Design review of the part built by this model. Coordinates are the model's own, in mm. Coordinates: 2 decimals unless noted, no trailing zeros. Loops run counter-clockwise (first coordinate to the right, second up) from the corner with the lowest first, then second, coordinate; pieces in that order, holes last. Notation, with made-up numbers: M 67.25,-5 L 108.25,-5 A20 ccw 108.25,27 Z; hole C 55.25,20.5 d2. An arc over 180 degrees is marked long. Answer as a JSON object with one key per item and string values. Group by question number.
1. Insertion check: pin 1 (4 mm diameter, centred on x = 64, z = 8.5, fed in from -Y); pin 2 (3.5 mm diameter, centred on y = -17, z = 7.5, fed in from -X) (3 decimals); pin 3 (0.5 mm diameter, centred on x = -104.5, y = -19, fed in from -Z). Each pin has a flat end and moves straight along its axis. Give the tip position at first contact, or say it passes through.
2. To check wall thickness, follow probe 1 along X at (y, z) = (-35, 7) (3 decimals); probe 2 along X at (y, z) = (-9.5, 2) (3 decimals); probe 3 along Y at (x, z) = (-87.5, 7) (1 decimal). State the ranges of each line that lie inside material, in increasing order.
3. Consider section A-A (z = 3.75). State the section outline as (x, y) points (3 decimals), then the cut area to 3 significant figures.
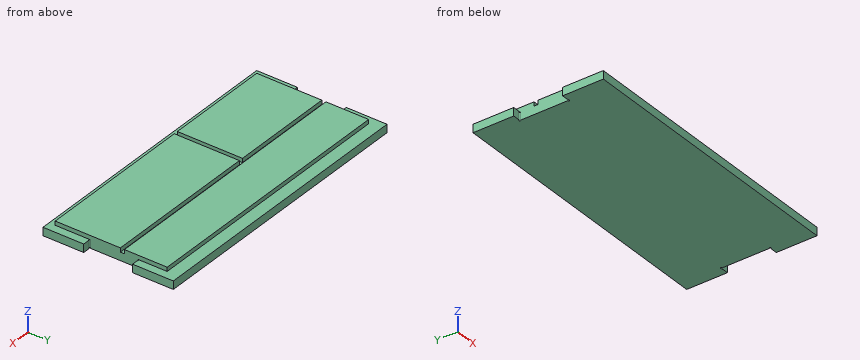
from build123d import *

# Parameters (mm, degrees)
F0_W     = 222.25
F0_H     = 101.6
F1_DEPTH = 9.525
F2_W     = 6.35
F2_H     = 38.1
F3_DEPTH = 9.526
F5_DEPTH = 3.175
F6_W     = 3.175
F6_H     = 50.8
F7_DEPTH = 3.175
F9_DEPTH = 6.35


with BuildPart() as f1:
    # F0 (on Top) → F1 (new body)
    with BuildSketch(Plane.XY):
        Rectangle(F0_W, F0_H)
    extrude(amount=F1_DEPTH)

    # F2 (on face) → F3 (cut, through all)
    with BuildSketch(Plane.XY.offset(9.525)):
        with Locations((-107.95, 0)):
            Rectangle(F2_W, F2_H)
        with Locations((107.95, 0)):
            Rectangle(F2_W, F2_H)
    extrude(amount=-F3_DEPTH, mode=Mode.SUBTRACT)

    # F4 (on face) → F5 (cut)
    with BuildSketch(Plane.XY.offset(9.525)):
        Polygon((-104.775, -46.0375), (-104.775, -19.05), (-111.125, -19.05), (-111.125, -50.8), (111.125, -50.8), (111.125, -19.05), (104.775, -19.05), (104.775, -46.0375), align=None)
        Polygon((-111.125, 19.05), (-104.775, 19.05), (-104.775, 41.275), (104.775, 41.275), (104.775, 19.05), (111.125, 19.05), (111.125, 50.8), (-111.125, 50.8), align=None)
    extrude(amount=-F5_DEPTH, mode=Mode.SUBTRACT)

    # F6 (on face) → F7 (cut)
    with BuildSketch(Plane.XY.offset(9.525)):
        Polygon((104.775, 7.9375), (-104.775, 7.9375), (-104.775, 4.7625), (-22.225, 4.7625), (-19.05, 4.7625), (104.775, 4.7625), align=None)
        with Locations((-20.6375, -20.6375)):
            Rectangle(F6_W, F6_H)
    extrude(amount=-F7_DEPTH, mode=Mode.SUBTRACT)

    # F8 (on face) → F9 (cut, through all)
    with BuildSketch(Plane(origin=(0, 0, 0), x_dir=(1, 0, 0), z_dir=(0, 0, -1))):
        with BuildLine():
            ThreePointArc((105.41, 19.05), (104.325987, 19.499013), (104.775, 18.415))
            Line((104.775, 18.415), (104.775, 19.05))
            Line((104.775, 19.05), (105.41, 19.05))
        make_face()
        with BuildLine():
            ThreePointArc((104.775, -18.415), (104.325987, -19.499013), (105.41, -19.05))
            Line((105.41, -19.05), (104.775, -19.05))
            Line((104.775, -19.05), (104.775, -18.415))
        make_face()
        with BuildLine():
            Line((-104.775, -19.05), (-105.41, -19.05))
            ThreePointArc((-105.41, -19.05), (-104.325987, -19.499013), (-104.775, -18.415))
            Line((-104.775, -18.415), (-104.775, -19.05))
        make_face()
        with BuildLine():
            Line((-104.775, 19.05), (-104.775, 18.415))
            ThreePointArc((-104.775, 18.415), (-104.325987, 19.499013), (-105.41, 19.05))
            Line((-105.41, 19.05), (-104.775, 19.05))
        make_face()
    extrude(amount=-F9_DEPTH, mode=Mode.SUBTRACT)


solid = f1.part
Findings below:
{
 "1": {"pin 1": "stops at y = -46.04", "pin 2": "stops at x = -104.775", "pin 3": "stops at z = 6.35"},
 "2": {"probe 1": "x = -104.775 to -22.225, -19.05 to 104.775", "probe 2": "x = -104.775 to 104.775", "probe 3": "y = -46 to 4.8, 7.9 to 41.3"},
 "3": {"outline": "M -111.125,-50.8 L 111.125,-50.8 L 111.125,-19.05 L 105.41,-19.05 A0.635 cw long 104.775,-18.415 L 104.775,18.415 A0.635 cw long 105.41,19.05 L 111.125,19.05 L 111.125,50.8 L -111.125,50.8 L -111.125,19.05 L -105.41,19.05 A0.635 cw long -104.775,18.415 L -104.775,-18.415 A0.635 cw long -105.41,-19.05 L -111.125,-19.05 Z", "area": "22,100 mm^2"}
}
